Read the model definition and answer for the solid it produces. Units are mm, in the model's axes. Coordinates: 2 decimals unless noted, no trailing zeros.
from build123d import *

# Parameters (mm, degrees)
SKETCH1_R           = 0.645583979
SKETCH1_R_2         = 0.656166882
SKETCH1_R_3         = 0.486835056
SKETCH1_R_4         = 1.5
BOSS_EXTRUDE1_DEPTH = 1.6


with BuildPart() as part:
    # Sketch1 → Boss-Extrude1 (new body)
    with BuildSketch(Plane(origin=(0, 0, 0), x_dir=(1, 0, 0), z_dir=(0, 1, 0))):
        with BuildLine():
            Line((35.009657829, 35.009663213), (-35.009668596, 35.009663213))
            Line((-35.009668596, 35.009663213), (-35.009668596, -35.009663213))
            Line((-35.009668596, -35.009663213), (35.009668596, -35.009663213))
            Line((35.009668596, -35.009663213), (35.009668596, -16.996819979))
            Line((35.009668596, -16.996819979), (34.988502791, -16.996830745))
            add(Edge.make_bspline(
                [(34.988502791, -16.996830745), (34.988502791, -15.896155035), (34.078330096, -15.007158911), (32.998830957, -15.007158912)],
                knots=[6, 6, 6, 6, 7, 7, 7, 7], degree=3))
            Line((32.998830957, -15.007158912), (32.977665152, -14.985993106))
            add(Edge.make_bspline(
                [(32.977665152, -14.985993106), (30.226002792, -14.985993106), (28.003507099, -12.742331608), (28.003507099, -9.990669248)],
                knots=[8, 8, 8, 8, 9, 9, 9, 9], degree=3))
            Line((28.003507099, -9.990669248), (28.003507099, 9.990669248))
            Line((28.003507099, 9.990669248), (28.003507099, 10.011835053))
            add(Edge.make_bspline(
                [(28.003507099, 10.011835053), (28.003507099, 12.784663218), (30.226002792, 15.007158911), (32.977675917, 15.007158911)],
                knots=[11, 11, 11, 11, 12, 12, 12, 12], degree=3))
            Line((32.977675917, 15.007158911), (32.99883634, 15.028319334))
            add(Edge.make_bspline(
                [(32.99883634, 15.028319334), (34.078335478, 15.028322254), (34.988494945, 15.938497412), (34.988492025, 17.017996551)],
                knots=[13, 13, 13, 13, 14, 14, 14, 14], degree=3))
            Line((34.988492025, 17.017996551), (35.00965783, 16.996830745))
            add(Edge.make_bspline(
                [(35.00965783, 16.996830745), (35.009657829, 35.009673979), (35.009657829, 35.009663213)],
                knots=[0, 0, 0, 1, 1, 1], degree=2))
        make_face()
        with Locations((-7.503590222, 31.517165368)):
            Circle(SKETCH1_R, mode=Mode.SUBTRACT)
        with Locations((-2.508255598, 31.517165368)):
            Circle(SKETCH1_R, mode=Mode.SUBTRACT)
        with Locations((2.487079026, 31.517165369)):
            Circle(SKETCH1_R, mode=Mode.SUBTRACT)
        with Locations((7.492996552, 31.517165369)):
            Circle(SKETCH1_R_2, mode=Mode.SUBTRACT)
        with Locations((-15.007175061, 28.215170536)):
            Circle(SKETCH1_R_3, mode=Mode.SUBTRACT)
        with Locations((-15.007175061, 32.004000424)):
            Circle(SKETCH1_R_3, mode=Mode.SUBTRACT)
        with Locations((1.989661068, 7.51416236)):
            Circle(SKETCH1_R_2, mode=Mode.SUBTRACT)
        with Locations((1.989661069, 2.518838502)):
            Circle(SKETCH1_R_2, mode=Mode.SUBTRACT)
        with Locations((1.989661069, -2.476496122)):
            Circle(SKETCH1_R_2, mode=Mode.SUBTRACT)
        with Locations((1.989661069, -7.492996551)):
            Circle(SKETCH1_R_2, mode=Mode.SUBTRACT)
        with Locations((-7.503590219, -31.474833755)):
            Circle(SKETCH1_R, mode=Mode.SUBTRACT)
        with Locations((-2.508255595, -31.474833755)):
            Circle(SKETCH1_R, mode=Mode.SUBTRACT)
        with Locations((2.487079029, -31.474833754)):
            Circle(SKETCH1_R, mode=Mode.SUBTRACT)
        with Locations((7.492996555, -31.474833754)):
            Circle(SKETCH1_R_2, mode=Mode.SUBTRACT)
        with Locations((-31.009175272, 31.009164506)):
            Circle(SKETCH1_R_4, mode=Mode.SUBTRACT)
        with Locations((30.9879987, 31.009164509)):
            Circle(SKETCH1_R_4, mode=Mode.SUBTRACT)
        with Locations((-31.009175269, -30.9879987)):
            Circle(SKETCH1_R_4, mode=Mode.SUBTRACT)
        with Locations((30.987998703, -30.987998698)):
            Circle(SKETCH1_R_4, mode=Mode.SUBTRACT)
        with Locations((14.985998491, -27.686003867)):
            Circle(SKETCH1_R_3, mode=Mode.SUBTRACT)
        with Locations((14.985998491, -31.495999559)):
            Circle(SKETCH1_R_3, mode=Mode.SUBTRACT)
    extrude(amount=BOSS_EXTRUDE1_DEPTH)


solid = part.part
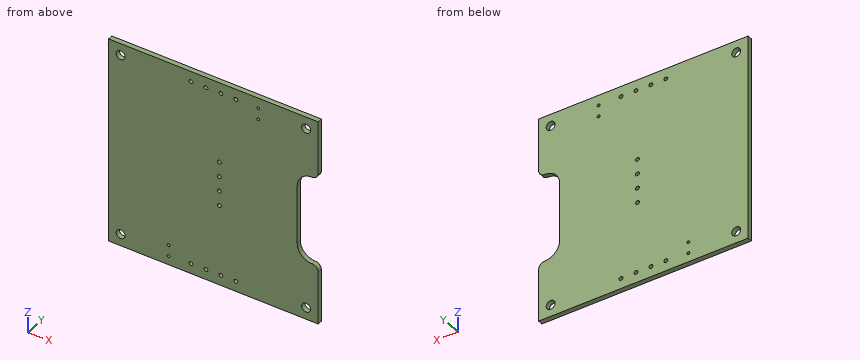
Item 1: Given pin 1 (1.5 mm diameter, centred on x = 7.49, z = -31.52, fed in from +Y), flat-ended and moving along its own axis, determine where the tip first touches the part or whether it passes through.
Numbers:
pin 1: stops at y = 1.6
Item 2: A cutting plane is placed at A-A on y = 0.7. Give the number of separate pieces and of enclosed holes in the cut face, then the cut area to 3 significant figures.
Numbers:
separate pieces: 1
enclosed holes: 20
area: 4,650 mm2
Item 3: Find the intervals of material crossed by line 1 along Z through (x, y) = (-30.5, 1.25); line 2 along X through (y, z) = (1.15, -3.5); line 3 along Z through (x, y) = (-3, 0.9), in increasing order.
Numbers:
line 1: z = -35.01 to -32.42, -29.6 to 29.58, 32.4 to 35.01
line 2: x = -35.01 to 28
line 3: z = -35.01 to -31.94, -31.1 to 31.06, 31.89 to 35.01
